```python
from build123d import *

# Parameters (mm, degrees)
F2_R    = 5
F3_R    = 30
F4_SIZE = 5


with BuildPart() as f1:
    # F0 (on Front) → F1 (revolve)
    with BuildSketch(Plane.XZ):
        Polygon((4, 20), (4, 0), (14, 0), (40, 40), (5, 30), (0, 30), (0, 25), align=None)
    revolve(axis=Axis((0, 0, 22.69237), (0, 0, 1)))

    # F2
    f2_edges = [f1.edges().sort_by_distance(p)[0] for p in [
        (-40, 0, 40),
    ]]
    fillet(f2_edges, radius=F2_R)

    # F3
    f3_edges = [f1.edges().sort_by_distance(p)[0] for p in [
        (-5, 0, 30),
    ]]
    fillet(f3_edges, radius=F3_R)

    # F4
    f4_edges = [f1.edges().sort_by_distance(p)[0] for p in [
        (-4, 0, 0),
    ]]
    chamfer(f4_edges, length=F4_SIZE)


solid = f1.part
```
Here's how the part is built. I have some questions about the finished solid (model axes, mm). A direction names the side the tool comes from. Round coordinates to 2 decimals unless told otherwise and drop trailing zeros. Order: outer loops, then holes, each group sorted by start corner. A loop starts at its lowest first (then second) coordinate and runs counter-clockwise, first axis right, second up. Notation, with made-up numbers: (85.25, 13) -> (100.25, 13) arc R13 cw to (100.25, 31) -> close; hole circle Ø9 at (-39, 35.25). An arc over 180 degrees is marked (long way). Use a Markdown table: item, result. Add a question column.
(1) For faces 1 (the face through (0, 0, 30)), 2 (the face through (-0.9, -4.1, 4.8)), which set-ups out of +Z, -Z, +X, -X, +Y, -Y let a thin tool reach every point of the face, with its end or its side?
(2) Suppose I cut it at B-B, the plane z = 26.5. Please give me the cut outline in (x, y) (3 decimals), and give its area (3 significant figures).
(3) For pin 1 Ø5 at (y, z) = (-6, 8) entering from +X; pin 2 Ø5 at (x, y) = (22.5, -20) entering from +Z; pin 3 Ø1.3 at (x, y) = (0, 0) entering from +Z; pin 4 Ø4 at (y, z) = (14.5, 12.5) entering from -X, each with a flat end and sliding along its axis, tell me the tip position at first contact or that it passes through.
(4) I need wall thicknesses on line 1 along Y through (x, z) = (0, 9.25); line 2 along Y through (x, z) = (0, 15.25); line 3 along Z through (x, y) = (5, -7.5). Which ranges of each line are inside material? Lowest first, please.
(5) Suppose I cut it at C-C, the plane z = 12.5. Please give me the cut outline in (x, y) (3 decimals).
(6) If we mould it in two halves opening along Y, with no side actions, what happens to faces 3 (the face through (16.454, 5.182, 5.001)), 4 (the face through (-0.867, -3.905, 12.395)), 5 (the face through (-9, -3, 0))? For each: released by +Y, released by -Y, zero draft, split by the parting line, or undercut.
(7) Suppose I cut it at A-A, the plane z = 17. Please give me the cut outline in (x, y).
Verdict:
| question | item | result |
|---|---|---|
| 1 | face 1 | +Z |
| 1 | face 2 | -Z |
| 2 | outline | circle Ø62.45 at (0, 0) |
| 2 | area | 3,060 mm2 |
| 3 | pin 1 | x = 20.08 |
| 3 | pin 2 | z = 36.52 |
| 3 | pin 3 | z = 30 |
| 3 | pin 4 | x = -18.97 |
| 4 | line 1 | -20.01 to -4, 4 to 20.01 |
| 4 | line 2 | -23.91 to -4, 4 to 23.91 |
| 4 | line 3 | 0 to 31.15 |
| 5 | outline | circle Ø44.25 at (0, 0); hole circle Ø8 at (0, 0) |
| 6 | face 3 | split by the parting line |
| 6 | face 4 | undercut |
| 6 | face 5 | zero draft |
| 7 | outline | circle Ø50.1 at (0, 0); hole circle Ø8 at (0, 0) |
